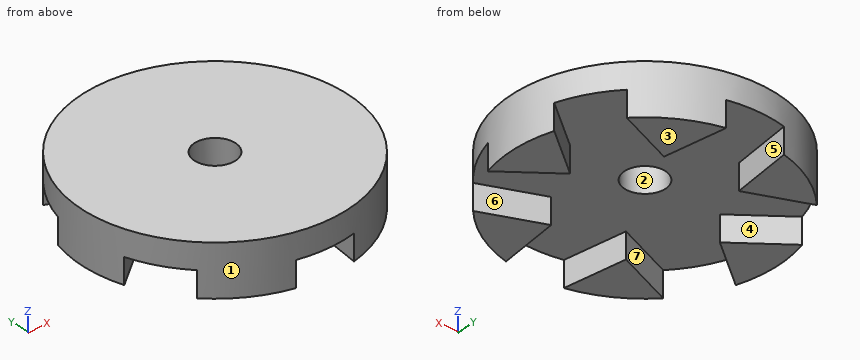
```python
from build123d import *

# Parameters (mm, degrees)
SKETCH_3_R          = 13
EXTRUDE_1_DEPTH     = 5
CUT_EXTRUDE_2_DEPTH = 2.5
SKETCH_6_R          = 2
CUT_EXTRUDE_3_DEPTH = 18
SKETCH_7_R          = 7.5
CUT_EXTRUDE_4_DEPTH = 8
CUT_EXTRUDE_6_DEPTH = 5
FILLET_1_R          = 1
SKETCH_10_W         = 2
SKETCH_10_H         = 13.5
CUT_EXTRUDE_7_DEPTH = 0.5
SKETCH_11_R         = 25
CUT_EXTRUDE_8_DEPTH = 13


with BuildPart() as part:
    # ｽｹｯﾁ3 → ﾎﾞｽ - 押し出し1 (new body)
    with BuildSketch(Plane.XY):
        Circle(SKETCH_3_R)
    extrude(amount=EXTRUDE_1_DEPTH)

    # ｽｹｯﾁ2 → ｶｯﾄ - 押し出し2 (cut)
    with BuildSketch(Plane.XY):
        with BuildLine():
            Line((3.75, 6.495190528), (2.773808556, 13.582081265))
            ThreePointArc((2.773808556, 13.582081265), (0, 16), (-2.773808556, 13.582081265))
            Line((-2.773808556, 13.582081265), (-3.75, 6.495190528))
            Line((-3.75, 6.495190528), (-10.375523134, 9.193229308))
            ThreePointArc((-10.375523134, 9.193229308), (-13.856406461, 8), (-13.14933169, 4.388851958))
            Line((-13.14933169, 4.388851958), (-7.5, 0))
            Line((-7.5, 0), (-13.14933169, -4.388851958))
            ThreePointArc((-13.14933169, -4.388851958), (-13.856406461, -8), (-10.375523134, -9.193229308))
            Line((-10.375523134, -9.193229308), (-3.75, -6.495190528))
            Line((-3.75, -6.495190528), (-2.773808556, -13.582081265))
            ThreePointArc((-2.773808556, -13.582081265), (0, -16), (2.773808556, -13.582081265))
            Line((2.773808556, -13.582081265), (3.75, -6.495190528))
            Line((3.75, -6.495190528), (10.375523134, -9.193229308))
            ThreePointArc((10.375523134, -9.193229308), (13.856406461, -8), (13.14933169, -4.388851958))
            Line((13.14933169, -4.388851958), (7.5, 0))
            Line((7.5, 0), (13.14933169, 4.388851958))
            ThreePointArc((13.14933169, 4.388851958), (13.856406461, 8), (10.375523134, 9.193229308))
            Line((10.375523134, 9.193229308), (3.75, 6.495190528))
        make_face()
    extrude(amount=CUT_EXTRUDE_2_DEPTH, mode=Mode.SUBTRACT)

    # ｽｹｯﾁ5 → 回転1 (revolve)
    with BuildSketch(Plane(origin=(0, 0, 0), x_dir=(1, 0, 0), z_dir=(0, 1, 0))):
        Polygon((0, -5), (25, -5), (25, -7), (10, -7), (10, -15), (25, -15), (25, -17), (0, -17), align=None)
    revolve(axis=Axis((0, 0, 0), (0, 0, 1)))

    # ｽｹｯﾁ6 → ｶｯﾄ - 押し出し3 (cut, through all)
    with BuildSketch(Plane.XY.offset(17)):
        Circle(SKETCH_6_R)
    extrude(amount=-CUT_EXTRUDE_3_DEPTH, mode=Mode.SUBTRACT)

    # ｽｹｯﾁ7 → ｶｯﾄ - 押し出し4 (cut)
    with BuildSketch(Plane.XY.offset(17)):
        Circle(SKETCH_7_R)
    extrude(amount=-CUT_EXTRUDE_4_DEPTH, mode=Mode.SUBTRACT)

    # ｽｹｯﾁ9 → ｶｯﾄ - 押し出し6 (cut)
    with BuildSketch(Plane(origin=(0, 0, 15), x_dir=(-1, 0, 0), z_dir=(0, 0, -1))):
        Polygon((-3.843473937, -0.691164305), (-11.556925253, -9.883697623), (-7.726703038, -13.097635671), (-0.013251721, -3.905102354), align=None)
    cut_extrude_6 = extrude(amount=CUT_EXTRUDE_6_DEPTH, mode=Mode.SUBTRACT)

    # ﾐﾗｰ1: ｶｯﾄ - 押し出し6 across plane
    add(cut_extrude_6.mirror(Plane(origin=(0, 0, 0), x_dir=(0, 0, 1), z_dir=(1, 0, 0))), mode=Mode.SUBTRACT)

    # ﾌｨﾚｯﾄ1
    fillet_1_edges = [part.edges().sort_by_distance(p)[0] for p in [
        (4.308653161, -9.024162451, 12.5),
        (-4.308653161, -9.024162451, 12.5),
    ]]
    fillet(fillet_1_edges, radius=FILLET_1_R)

    # ｽｹｯﾁ10 → ｶｯﾄ - 押し出し7 (cut)
    with BuildSketch(Plane.XY.offset(17)):
        with Locations((0, 16.25)):
            Rectangle(SKETCH_10_W, SKETCH_10_H)
    extrude(amount=-CUT_EXTRUDE_7_DEPTH, mode=Mode.SUBTRACT)

    # ｽｹｯﾁ11 → ｶｯﾄ - 押し出し8 (cut, through all)
    with BuildSketch(Plane(origin=(0, 0, 5), x_dir=(-1, 0, 0), z_dir=(0, 0, -1))):
        Circle(SKETCH_11_R)
    extrude(amount=-CUT_EXTRUDE_8_DEPTH, mode=Mode.SUBTRACT)


solid = part.part
```
CAD build for the part. Positions are in the model's coordinates, mm. Face numbers are marked on the shaded views. A direction names the side the tool comes from. Round coordinates to 2 decimals unless told otherwise and drop trailing zeros. Loops run counter-clockwise (first coordinate to the right, second up) from the corner with the lowest first, then second, coordinate; pieces in that order, holes last. Notation, with made-up numbers: M 86.5,-5 L 97.5,-5 A30 ccw 97.5,31 Z; hole C 46.5,9 d6. An arc over 180 degrees is marked long. Use a Markdown table: item, result. Add a question column.
(1) Which spindle directions (+Z, -Z, +X, -X, +Y, -Y) get a long thin tool onto all of the face, cutting with end or side? Do the marked faces 5, 6 and 7. Say none if no direction does.
(2) Drill centre lines: line 1 (Y direction, x = 0, z = 4.2); line 2 (Y direction, x = 9.25, z = 2.35); line 3 (Y direction, x = 7.75, z = 0.6). Where is each one in solid material? Low to high.
(3) Cut at C-C (y = -1.5). Give the cut face in (x, z), and give its area (3 significant figures).
(4) Flat gauge pins, fed straight in: pin 1 (1 mm diameter, centred on y = -9, z = 0.5, fed in from +X); pin 2 (1 mm diameter, centred on x = -7.5, z = 1.5, fed in from -Y). Where does each tip first touch, or does it go through?
(5) Cut at D-D (z = 3.9). Give the cut face in (x, y), and give its area (3 significant figures).
(6) Cut at A-A (z = 0.75). Give the cut face in (x, y).
(7) Pull direction X, two halves, no side cores. Call the marked faces 1, 2, 3 and 4: +X half, -X half, draft (parallel to the pull), parting line (faces both ways), or undercut.
(8) Cut at B-B (x = 0). Give the cut face in (y, z).
Geometry says:
| question | item | result |
|---|---|---|
| 1 | face 5 | -Z |
| 1 | face 6 | -Z, +X |
| 1 | face 7 | -Z, -X |
| 2 | line 1 | y = -13 to -2, 2 to 13 |
| 2 | line 2 | y = -9.13 to -8.73, -1.36 to 1.36, 8.73 to 9.13 |
| 2 | line 3 | y = -10.44 to -8.12, -0.19 to 0.19, 8.12 to 10.44 |
| 3 | outline | M -12.91,0 L -9.43,0 L -9.43,2.5 L -1.32,2.5 L -1.32,5 L -12.91,5 Z; M 1.32,2.5 L 9.43,2.5 L 9.43,0 L 12.91,0 L 12.91,5 L 1.32,5 Z |
| 3 | area | 75.4 mm² |
| 4 | pin 1 | stops at x = 9.53 |
| 4 | pin 2 | stops at y = -10.95 |
| 5 | outline | C 0,0 d26; hole C 0,0 d4 |
| 5 | area | 518 mm² |
| 6 | outline | M -12.42,-3.83 L -7.5,0 L -12.42,3.83 A13 ccw Z; M -9.53,-8.85 A13 ccw -2.9,-12.67 L -3.75,-6.5 Z; M -9.53,8.85 L -3.75,6.5 L -2.9,12.67 A13 ccw Z; M 2.9,-12.67 A13 ccw 9.53,-8.85 L 3.75,-6.5 Z; M 2.9,12.67 L 3.75,6.5 L 9.53,8.85 A13 ccw Z; M 7.5,0 L 12.42,-3.83 A13 ccw 12.42,3.83 Z |
| 7 | face 1 | parting line |
| 7 | face 2 | undercut |
| 7 | face 3 | draft |
| 7 | face 4 | undercut |
| 8 | outline | M -13,2.5 L -2,2.5 L -2,5 L -13,5 Z; M 2,2.5 L 13,2.5 L 13,5 L 2,5 Z |
